Autodesk Inventor part; units mm, degrees
ref_plane "YZ Plane" through (0, 0, 0) normal (1, 0, 0) x (0, 1, 0)
ref_plane "XZ Plane" through (0, 0, 0) normal (0, 1, 0) x (-1, 0, 0)
ref_plane "XY Plane" through (0, 0, 0) normal (0, 0, 1) x (1, 0, 0)
sketch "Sketch1" plane through (0, 0, 0) normal (0, 0, 1) x (1, 0, 0)
  circle A0 centre (0, 0) radius 6.35
  line L0 (7.3298, -0.1918) -> (3.4988, -6.4437)
  line L1 (3.4988, -6.4437) -> (-3.831, -6.2519)
  line L2 (-3.831, -6.2519) -> (-7.3298, 0.1918)
  line L3 (-7.3298, 0.1918) -> (-3.4988, 6.4437)
  line L4 (-3.4988, 6.4437) -> (3.831, 6.2519)
  line L5 (3.831, 6.2519) -> (7.3298, -0.1918)
  circle A1 centre (0, 0) radius 12.7
  point P0 (5.5804, 3.0301)
  dimension "d0" = 12.7
  dimension "d1" = 25.4
extrude "Extrusion1" add sketch "Sketch1" along normal blind 25.4
properties part number "4-bar intake (1'') spacer"
Work out the finished part from the listing and answer in its coordinate system (mm). Coordinates: 2 decimals unless noted, no trailing zeros. Loops run counter-clockwise (first coordinate to the right, second up) from the corner with the lowest first, then second, coordinate; pieces in that order, holes last. Notation, with made-up numbers: (85.25, 19.25) -> (116.25, 19.25) arc R38 ccw to (116.25, 58.25) -> close; hole circle Ø8 at (-12, -35). An arc over 180 degrees is marked (long way). Answer as CSV lines item,"result".
Q1. The part is cut by section C-C on y = -5.5. Write down the section's boundary in (x, z).
Findings:
outline,"(-11.45, 0) -> (-4.24, 0) -> (-4.24, 25.4) -> (-11.45, 25.4) -> close; (4.08, 0) -> (11.45, 0) -> (11.45, 25.4) -> (4.08, 25.4) -> close"
Q2. The part is cut by section D-D on x = 10.25. Write down the section's boundary in (y, z).
Findings:
outline,"(-7.5, 0) -> (7.5, 0) -> (7.5, 25.4) -> (-7.5, 25.4) -> close"
Q3. Find the intervals of material crossed by probe 1 along X at (y, z) = (-4.75, 18.75); probe 2 along X at (y, z) = (0.5, 12); probe 3 along Y at (x, z) = (11, 5), in increasing order.
Findings:
probe 1,"x = -11.78 to -4.65, 4.54 to 11.78"
probe 2,"x = -12.69 to -7.14, 6.95 to 12.69"
probe 3,"y = -6.35 to 6.35"
Q4. The part is cut by section B-B on x = -1.75. Write down the section's boundary in (y, z), and give its area (3 significant figures).
Findings:
outline,"(-12.58, 0) -> (-6.31, 0) -> (-6.31, 25.4) -> (-12.58, 25.4) -> close; (6.4, 0) -> (12.58, 0) -> (12.58, 25.4) -> (6.4, 25.4) -> close"
area,"316 mm²"
Q5. Each of these flat-tipped pins is pushed along its axis until it touches: pin 1 (2 mm diameter, centred on x = 8, z = 9.5, fed in from -Y); pin 2 (5 mm diameter, centred on x = 0.5, y = -3.5, fed in from -Z); pin 3 (1.5 mm diameter, centred on y = 5.5, z = 10, fed in from +X); pin 4 (1 mm diameter, centred on y = 5, z = 6.5, fed in from +X). Where does it stop, or does it pass through?
Findings:
pin 1,"stops at y = -10.6"
pin 2,"passes through"
pin 3,"stops at x = 11.78"
pin 4,"stops at x = 11.88"
Q6. The part is cut by section A-A on z = 8.5. Write down the section's boundary in (x, y), and give its area (3 significant figures).
Findings:
outline,"circle Ø25.4 at (0, 0); hole (-7.33, 0.19) -> (-3.83, -6.25) -> (3.5, -6.44) -> (7.33, -0.19) -> (3.83, 6.25) -> (-3.5, 6.44) -> close"
area,"367 mm²"
